Part model, mm, in its own coordinate system. Face numbers are marked on the shaded views. Round coordinates to 2 decimals unless told otherwise and drop trailing zeros. Write each loop counter-clockwise with the first axis right and the second up, starting at its lowest first coordinate (ties: lowest second). Pieces come first, ordered by that corner, then holes. Notation, with made-up numbers: M 6,-10 L 21,-10 A36 ccw 21,26 Z; hole C -17.5,36.25 d6. An arc over 180 degrees is marked long. Use one line per item in the form item = value. Start each with the question number.
Item 1: Flat gauge pins, fed straight in: pin 1 Ø1 at (y, z) = (-20.5, 21.5) entering from -X; pin 2 Ø5 at (x, z) = (-44, 96.5) entering from +Y; pin 3 Ø12 at (x, z) = (51, 29.5) entering from -Y. Where does each tip first touch, or does it go through?
Item 2: Cut at D-D, the plane x = -47.5. Give the cut face in (y, z), then the cut area to 3 significant figures.
Item 3: Mould opens along Y. For the marked faces 1, 2 and 3 say: +Y half, -Y half, draft (parallel to the pull), parting line (faces both ways), or undercut.
Item 4: Cut at C-C, the plane z = 46. Give the cut face in (x, y), then the cut area to 3 significant figures.
Item 5: Probe L1, parallel to Y at x = 0, z = 3; L2, parallel to X at y = 7, z = 9; L3, parallel to Z at x = 44.5, y = 15. List the from-to ranges inside material, lowest first.
Item 6: Cut at A-A, the plane y = 0. Give the cut face in (x, z), then the cut area to 3 significant figures.
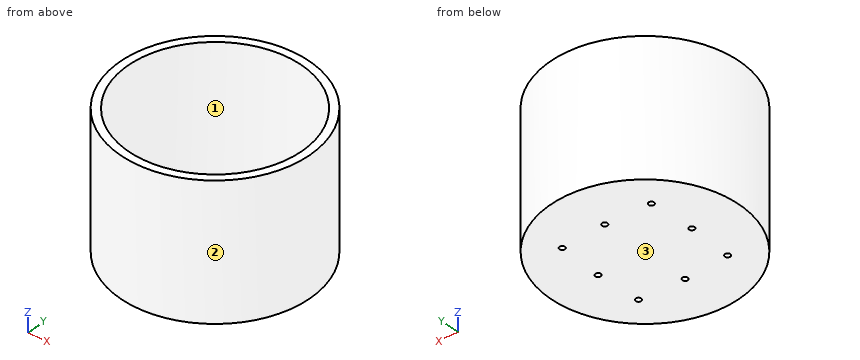
from build123d import *

# Parameters (mm, degrees)
SKETCH1_R           = 76.2
SKETCH1_R_2         = 69.85
BOSS_EXTRUDE1_DEPTH = 107.95
SKETCH3_R           = 76.2
BOSS_EXTRUDE2_DEPTH = 6.35
SKETCH5_R           = 2.1828125
CUT_EXTRUDE2_DEPTH  = 7.35
SKETCH11_R          = 2.1828125
CUT_EXTRUDE11_DEPTH = 7.35
SKETCH4_3_W         = 38.1
SKETCH4_3_H         = 38.1
BOSS_EXTRUDE3_DEPTH = 19.05


with BuildPart() as part:
    # Sketch1 → Boss-Extrude1 (new body)
    with BuildSketch(Plane.XY):
        Circle(SKETCH1_R)
        Circle(SKETCH1_R_2, mode=Mode.SUBTRACT)
    extrude(amount=BOSS_EXTRUDE1_DEPTH)

    # Sketch3 → Boss-Extrude2 (add)
    with BuildSketch(Plane.XY):
        Circle(SKETCH3_R)
    extrude(amount=BOSS_EXTRUDE2_DEPTH)

    # Sketch5 → Cut-Extrude2 (cut, through all)
    with BuildSketch(Plane.XY.offset(6.35)):
        with Locations((0, 37.81298)):
            Circle(SKETCH5_R)
        with Locations((37.81298, 0)):
            Circle(SKETCH5_R)
        with Locations((-37.81298, 0)):
            Circle(SKETCH5_R)
        with Locations((0, -37.81298)):
            Circle(SKETCH5_R)
    extrude(amount=-CUT_EXTRUDE2_DEPTH, mode=Mode.SUBTRACT)

    # Sketch11 → Cut-Extrude11 (cut, through all)
    with BuildSketch(Plane.XY.offset(6.35)):
        with Locations((-35.921024484, 35.921024484)):
            Circle(SKETCH11_R)
        with Locations((-35.921024484, -35.921024484)):
            Circle(SKETCH11_R)
        with Locations((35.921024484, -35.921024484)):
            Circle(SKETCH11_R)
        with Locations((35.921024484, 35.921024484)):
            Circle(SKETCH11_R)
    extrude(amount=-CUT_EXTRUDE11_DEPTH, mode=Mode.SUBTRACT)

    # Sketch4_3 → Boss-Extrude3 (add)
    with BuildSketch(Plane.XY.offset(6.35)):
        Rectangle(SKETCH4_3_W, SKETCH4_3_H)
    extrude(amount=BOSS_EXTRUDE3_DEPTH)


solid = part.part
Model answer:
q1.pin_1 = -73.53
q1.pin_2 = 63.91
q1.pin_3 = -61.49
q2.outline = M -59.58,0 L 59.58,0 L 59.58,107.95 L 51.21,107.95 L 51.21,6.35 L -51.21,6.35 L -51.21,107.95 L -59.58,107.95 Z
q2.area = 2,460 mm²
q3.face_1 = undercut
q3.face_2 = parting line
q3.face_3 = draft
q4.outline = C 0,0 d152.4; hole C 0,0 d139.7
q4.area = 2,910 mm²
q5.L1 = -76.2 to -40, -35.63 to 35.63, 40 to 76.2
q5.L2 = -75.88 to -69.5, -19.05 to 19.05, 69.5 to 75.88
q5.L3 = 0 to 6.35
q6.outline = M -76.2,0 L -40,0 L -40,6.35 L -69.85,6.35 L -69.85,107.95 L -76.2,107.95 Z; M -35.63,0 L 35.63,0 L 35.63,6.35 L 19.05,6.35 L 19.05,25.4 L -19.05,25.4 L -19.05,6.35 L -35.63,6.35 Z; M 40,0 L 76.2,0 L 76.2,107.95 L 69.85,107.95 L 69.85,6.35 L 40,6.35 Z
q6.area = 2,930 mm²
